from build123d import *

# Parameters (mm, degrees)
F1_DEPTH = 43
F3_DEPTH = 28
F4_W     = 123
F4_H     = 12.5
F5_DEPTH = 39
F6_W     = 98
F6_H     = 4
F7_DEPTH = 38
F8_W     = 123
F8_H     = 20.5
F9_DEPTH = 39


with BuildPart() as f1:
    # F0 (on Top) → F1 (new body)
    with BuildSketch(Plane.XY):
        Polygon((-65.5, 0), (0, 0), (65.5, 0), (65.5, 45), (0, 45), (-65.5, 45), align=None)
    extrude(amount=-F1_DEPTH)

    # F2 (on face) → F3 (cut)
    with BuildSketch(Plane.XY):
        Polygon((-49, 4), (-49, 0), (0, 0), (49, 0), (49, 4), (0, 4), align=None)
    extrude(amount=-F3_DEPTH, mode=Mode.SUBTRACT)

    # F4 (on face) → F5 (cut)
    with BuildSketch(Plane.XY):
        with Locations((0, 10.25)):
            Rectangle(F4_W, F4_H)
    extrude(amount=-F5_DEPTH, mode=Mode.SUBTRACT)

    # F6 (on face) → F7 (cut)
    with BuildSketch(Plane.XY):
        with Locations((0, 18.5)):
            Rectangle(F6_W, F6_H)
    extrude(amount=-F7_DEPTH, mode=Mode.SUBTRACT)

    # F8 (on face) → F9 (cut)
    with BuildSketch(Plane.XY):
        with Locations((0, 30.75)):
            Rectangle(F8_W, F8_H)
    extrude(amount=-F9_DEPTH, mode=Mode.SUBTRACT)


solid = f1.part
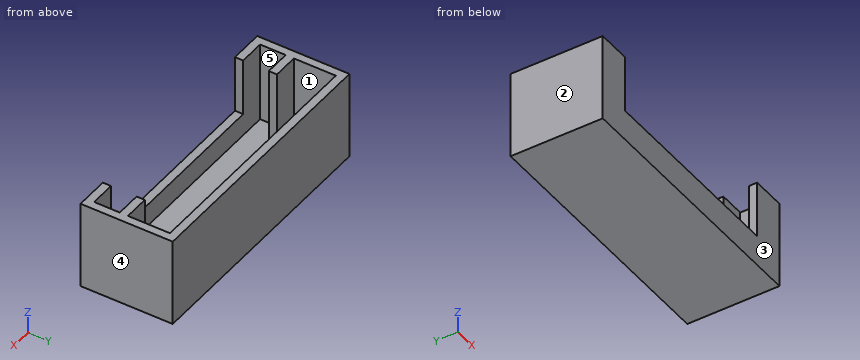
Input: part model. Units: mm. Frame: model coordinates. Face numbers are marked on the shaded views. A direction names the side the tool comes from. Coordinates: 2 decimals unless noted, no trailing zeros. Loops run counter-clockwise (first coordinate to the right, second up) from the corner with the lowest first, then second, coordinate; pieces in that order, holes last. Notation, with made-up numbers: (74, 34.5) - (84, 34.5) arc R16 ccw to (84, 39.5) - close; hole circle Ø4 at (43, 35). An arc over 180 degrees is marked (long way). Answer in a Markdown table with one row per item. Add a question column.
Item 1: Section query B-B on x = 38. Return the cut outline in (y, z), then the cut area to 3 significant figures.
Item 2: Contact query for flat-ended pins moving along their axis: P1, Ø3, axis at x = -17.5, y = 19.5, coming from the +Z side; P2, Ø1.2, axis at x = 6.5, y = 1, coming from the +Z side; P3, Ø2, axis at x = -21.5, y = 28.5, coming from the +Z side. Output: stop coordinate, or through.
Item 3: Access query for the marked faces 1 and 2. Directions: +Z, -Z, +X, -X, +Y, -Y. A direction counts if a zero-diameter tool reaches every point of the face in a straight line with its end or side. Return the directions, or none.
Item 4: Section query A-A on z = -35. Return the cut outline in (x, y).
Item 5: Line query: line 1 along Y through (x, z) = (-57, -30); line 2 along X through (y, z) = (22, -8.5); line 3 along Y through (x, z) = (24, -34). Output: solid intervals per line, ascending. Write a range as [from, to].
Item 6: Mould query, pull axis X, two halves, no side actions, for the marked faces 3, 4 and 5. Classes: released by +X, released by -X, zero draft, split by the parting line, or undercut.
Item 7: Section query C-C on y = 13. Return the cut outline in (x, z), then the cut area to 3 significant figures.
Item 8: Section query D-D on z = -12. Return the cut outline in (x, y).
Recorded:
| question | item | result |
|---|---|---|
| 1 | outline | (0, -43) - (45, -43) - (45, 0) - (41, 0) - (41, -39) - (20.5, -39) - (20.5, -38) - (16.5, -38) - (16.5, -39) - (4, -39) - (4, -28) - (0, -28) - close |
| 1 | area | 384 mm^2 |
| 2 | P1 | z = -38 |
| 2 | P2 | z = -28 |
| 2 | P3 | z = -39 |
| 3 | face 1 | +Z |
| 3 | face 2 | +Z, -Z, -X, +Y, -Y |
| 4 | outline | (-65.5, 0) - (65.5, 0) - (65.5, 45) - (-65.5, 45) - close; hole (-61.5, 4) - (61.5, 4) - (61.5, 16.5) - (49, 16.5) - (49, 20.5) - (61.5, 20.5) - (61.5, 41) - (-61.5, 41) - (-61.5, 20.5) - (-49, 20.5) - (-49, 16.5) - (-61.5, 16.5) - close |
| 5 | line 1 | [0, 4], [16.5, 20.5], [41, 45] |
| 5 | line 2 | [-65.5, -61.5], [61.5, 65.5] |
| 5 | line 3 | [0, 4], [41, 45] |
| 6 | face 3 | zero draft |
| 6 | face 4 | released by +X |
| 6 | face 5 | undercut |
| 7 | outline | (-65.5, -43) - (65.5, -43) - (65.5, 0) - (61.5, 0) - (61.5, -39) - (-61.5, -39) - (-61.5, 0) - (-65.5, 0) - close |
| 7 | area | 836 mm^2 |
| 8 | outline | (-65.5, 0) - (-49, 0) - (-49, 4) - (-61.5, 4) - (-61.5, 16.5) - (-49, 16.5) - (-49, 20.5) - (-61.5, 20.5) - (-61.5, 41) - (61.5, 41) - (61.5, 20.5) - (49, 20.5) - (49, 16.5) - (61.5, 16.5) - (61.5, 4) - (49, 4) - (49, 0) - (65.5, 0) - (65.5, 45) - (-65.5, 45) - close |
